Here's how the part is built. I have some questions about the finished solid (model axes, mm). Face numbers are marked on the shaded views. Round coordinates to 2 decimals unless told otherwise and drop trailing zeros. Loops run counter-clockwise (first coordinate to the right, second up) from the corner with the lowest first, then second, coordinate; pieces in that order, holes last. Notation, with made-up numbers: M -0.75,35.25 L 12.25,35.25 A27 ccw 12.25,74.25 Z; hole C -17,54.5 d7. An arc over 180 degrees is marked long. Answer as a JSON object with one key per item and string values.
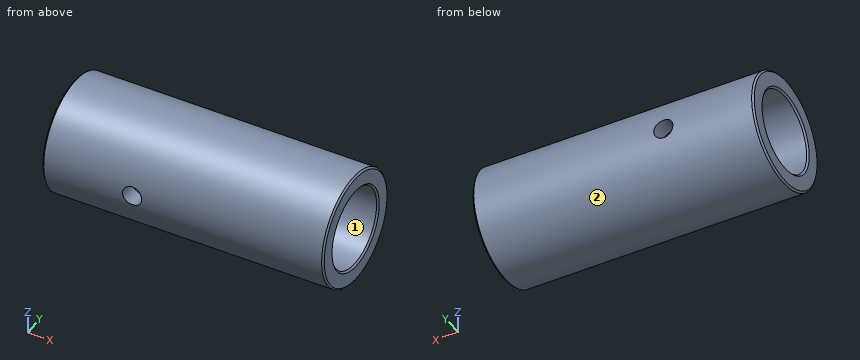
from build123d import *

# Parameters (mm, degrees)
SKETCH_1_R          = 50
SKETCH_1_R_2        = 35
EXTRUDE_1_DEPTH     = 250
SKETCH_2_R          = 8.5
CUT_EXTRUDE_1_DEPTH = 430
CHAMFER_1_SIZE      = 1.5


with BuildPart() as part:
    # Sketch 1 → Extrude 1 (new body)
    with BuildSketch(Plane(origin=(0, 0, 0), x_dir=(0, 0, -1), z_dir=(1, 0, 0))):
        Circle(SKETCH_1_R)
        Circle(SKETCH_1_R_2, mode=Mode.SUBTRACT)
    extrude(amount=EXTRUDE_1_DEPTH)

    # Sketch 2 → Cut-Extrude 1 (cut, symmetric)
    with BuildSketch(Plane(origin=(0, 0, 0), x_dir=(1, 0, 0), z_dir=(0, 1, 0))):
        with Locations(Location((80, 0, 0), (0, 0, 270))):
            Circle(SKETCH_2_R)
    extrude(amount=CUT_EXTRUDE_1_DEPTH, both=True, mode=Mode.SUBTRACT)

    # Chamfer 1
    chamfer_1_edges = [part.edges().sort_by_distance(p)[0] for p in [
        (0, 0, 50),
        (250, 0, 50),
        (0, 0, 35),
        (250, 0, 35),
    ]]
    chamfer(chamfer_1_edges, length=CHAMFER_1_SIZE)


solid = part.part
Item 1: I want a section at A-A on y = 0. List the corners of the cut face in (x, z) for me.
Solution:
{"outline": "M 0,-48.5 L 1.5,-50 L 248.5,-50 L 250,-48.5 L 250,-36.5 L 248.5,-35 L 1.5,-35 L 0,-36.5 Z; M 0,36.5 L 1.5,35 L 248.5,35 L 250,36.5 L 250,48.5 L 248.5,50 L 1.5,50 L 0,48.5 Z"}
Item 2: For P1, Ø4, axis at x = 213.5, y = -16.5, coming from the -Z side; P2, Ø3, axis at x = 172, z = 12, coming from the +Y side; P3, Ø6, axis at x = 52.5, y = -19, coming from the +Z side, each with a flat end and sliding along its axis, tell me the tip position at first contact or that it passes through.
Solution:
{"P1": "stops at z = -47.85", "P2": "stops at y = 48.89", "P3": "stops at z = 47.37"}
Item 3: If I drill on L1, parallel to X at y = -40.75, z = 0; L2, parallel to Y at x = 147, z = 0; L3, parallel to Y at x = 81, z = 21, over which ranges is the centre line in solid material (lowest first)? Write a range as from..to.
Solution:
{"L1": "x = 0..71.5, 88.5..250", "L2": "y = -50..-35, 35..50", "L3": "y = -45.38..-28, 28..45.38"}
Item 4: We'd pull the mould along Y, two halves only. Please class the marked faces 1 and 2: +Y half, -Y half, draft (parallel to the pull), parting line (faces both ways), or undercut.
Solution:
{"face 1": "undercut", "face 2": "parting line"}
Item 5: I want a section at C-C on x = 80. List the corners of the cut face in (y, z) for me.
Solution:
{"outline": "M -49.27,-8.5 A50 ccw 49.27,-8.5 L 33.95,-8.5 A35 cw -33.95,-8.5 Z; M -49.27,8.5 L -33.95,8.5 A35 cw 33.95,8.5 L 49.27,8.5 A50 ccw Z"}
Item 6: I want a section at B-B on z = 0. List the corners of the cut face in (x, y) for me.
Solution:
{"outline": "M 0,-48.5 L 1.5,-50 L 71.5,-50 L 71.5,-35 L 1.5,-35 L 0,-36.5 Z; M 0,36.5 L 1.5,35 L 71.5,35 L 71.5,50 L 1.5,50 L 0,48.5 Z; M 88.5,-50 L 248.5,-50 L 250,-48.5 L 250,-36.5 L 248.5,-35 L 88.5,-35 Z; M 88.5,35 L 248.5,35 L 250,36.5 L 250,48.5 L 248.5,50 L 88.5,50 Z"}
